from build123d import *

# Parameters (mm, degrees)
BOSS_EXTRUDE1_DEPTH = 4


with BuildPart() as part:
    # Sketch1 → Boss-Extrude1 (new body)
    with BuildSketch(Plane.XY):
        with BuildLine():
            ThreePointArc((2.5, -15), (15, -2.5), (27.5, -15))
            Line((27.5, -15), (30, -15))
            Line((30, -15), (30, 0))
            Line((30, 0), (0, 0))
            Line((0, 0), (0, -15))
            Line((0, -15), (2.5, -15))
        make_face()
        with BuildLine():
            Line((30, -15), (27.5, -15))
            ThreePointArc((27.5, -15), (15, -27.5), (2.5, -15))
            Line((2.5, -15), (0, -15))
            Line((0, -15), (0, -30))
            Line((0, -30), (30, -30))
            Line((30, -30), (30, -15))
        make_face()
        with BuildLine():
            ThreePointArc((23, -15), (25, -13), (27, -15))
            Line((27, -15), (27.5, -15))
            ThreePointArc((27.5, -15), (15, -2.5), (2.5, -15))
            Line((2.5, -15), (3, -15))
            ThreePointArc((3, -15), (5, -13), (7, -15))
            Line((7, -15), (13.5, -15))
            ThreePointArc((13.5, -15), (15, -13.5), (16.5, -15))
            Line((16.5, -15), (23, -15))
        make_face()
        with BuildLine():
            Line((27.5, -15), (27, -15))
            ThreePointArc((27, -15), (25, -17), (23, -15))
            Line((23, -15), (16.5, -15))
            ThreePointArc((16.5, -15), (15, -16.5), (13.5, -15))
            Line((13.5, -15), (7, -15))
            ThreePointArc((7, -15), (5, -17), (3, -15))
            Line((3, -15), (2.5, -15))
            ThreePointArc((2.5, -15), (15, -27.5), (27.5, -15))
        make_face()
    extrude(amount=BOSS_EXTRUDE1_DEPTH)


solid = part.part
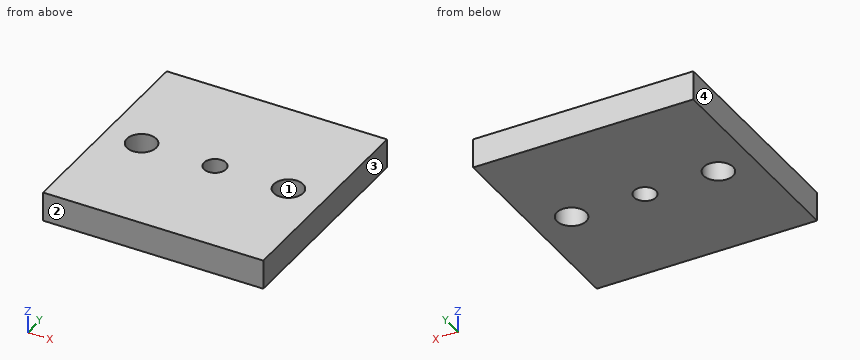
Model file for the job. Use its own axes, mm. Face numbers are marked on the shaded views. Round coordinates to 2 decimals unless told otherwise and drop trailing zeros. Order: outer loops, then holes, each group sorted by start corner. A loop starts at its lowest first (then second) coordinate and runs counter-clockwise, first axis right, second up.
(1) Band-saw the part on D-D (x = 25). List the corners of the cut face in (y, z), then the cut area to 3 significant figures.
(2) Pin check, flat tips, straight feed: pin 1 (5 mm diameter, centred on x = 17, y = -25, fed in from -Z); pin 2 (2.5 mm diameter, centred on x = 25, y = -15, fed in from +Z). Stop position of each tip, or through.
(3) Band-saw the part on B-B (z = 3). List the corners of the cut face in (x, y), then the cut area to 3 significant figures.
(4) Pull direction X, two halves, no side cores. Call the marked faces 1, 2, 3 and 4: released by +X, released by -X, zero draft, split by the parting line, or undercut.
(5) Band-saw the part on C-C (y = -14). List the corners of the cut face in (x, z).
(6) Drill centre lines: line 1 (X direction, y = -15, z = 1.9); line 2 (Y direction, x = 15, z = 1.85); line 3 (Y direction, x = 25, z = 1.9). Where is each one in solid material? Low to high.
(7) Band-saw the part on A-A (x = 15). List the corners of the cut face in (y, z).
Verdict:
1. outline: (-30, 0) - (-17, 0) - (-17, 4) - (-30, 4) - close; (-13, 0) - (0, 0) - (0, 4) - (-13, 4) - close
1. area: 104 mm2
2. pin 1: stops at z = 0
2. pin 2: passes through
3. outline: (0, -30) - (30, -30) - (30, 0) - (0, 0) - close; hole circle Ø4 at (5, -15); hole circle Ø3 at (15, -15); hole circle Ø4 at (25, -15)
3. area: 868 mm2
4. face 1: undercut
4. face 2: zero draft
4. face 3: released by +X
4. face 4: released by -X
5. outline: (0, 0) - (3.27, 0) - (3.27, 4) - (0, 4) - close; (6.73, 0) - (13.88, 0) - (13.88, 4) - (6.73, 4) - close; (16.12, 0) - (23.27, 0) - (23.27, 4) - (16.12, 4) - close; (26.73, 0) - (30, 0) - (30, 4) - (26.73, 4) - close
6. line 1: x = 0 to 3, 7 to 13.5, 16.5 to 23, 27 to 30
6. line 2: y = -30 to -16.5, -13.5 to 0
6. line 3: y = -30 to -17, -13 to 0
7. outline: (-30, 0) - (-16.5, 0) - (-16.5, 4) - (-30, 4) - close; (-13.5, 0) - (0, 0) - (0, 4) - (-13.5, 4) - close
